```python
from build123d import *

# Parameters (mm, degrees)
ESBO_O2_W                = 8
ESBO_O2_H                = 12
RESSALTO_EXTRUS_O1_DEPTH = 17
ESBO_O3_W                = 6.2
ESBO_O3_H                = 10.2
CORTE_EXTRUS_O1_DEPTH    = 15
ESBO_O4_R                = 12.5
RESSALTO_EXTRUS_O2_DEPTH = 12
ESBO_O5_R                = 11.5
CORTE_EXTRUS_O2_DEPTH    = 10


with BuildPart() as part:
    # Esboço2 → Ressalto-extrusão1 (new body)
    with BuildSketch(Plane.XY):
        Rectangle(ESBO_O2_W, ESBO_O2_H)
    extrude(amount=RESSALTO_EXTRUS_O1_DEPTH)

    # Esboço3 → Corte-extrusão1 (cut)
    with BuildSketch(Plane.XY.offset(17)):
        Rectangle(ESBO_O3_W, ESBO_O3_H)
    extrude(amount=-CORTE_EXTRUS_O1_DEPTH, mode=Mode.SUBTRACT)

    # Esboço4 → Ressalto-extrusão2 (add)
    with BuildSketch(Plane(origin=(0, 6, 0), x_dir=(1, 0, 0), z_dir=(0, 1, 0))):
        with Locations((0, 11.842719282)):
            Circle(ESBO_O4_R)
    extrude(amount=-RESSALTO_EXTRUS_O2_DEPTH)

    # Esboço5 → Corte-extrusão2 (cut)
    with BuildSketch(Plane(origin=(0, 6, 0), x_dir=(1, 0, 0), z_dir=(0, 1, 0))):
        with Locations(Location((0, 11.842719282, 0), (0, 0, 180))):
            Circle(ESBO_O5_R)
    extrude(amount=-CORTE_EXTRUS_O2_DEPTH, mode=Mode.SUBTRACT)


solid = part.part
```
Check sheet for the modelled part. Datum: model origin and axes. Units: mm. A direction names the side the tool comes from. Give positions to 0.01 mm unless a question says otherwise; leave off trailing zeros. Write each loop counter-clockwise with the first axis right and the second up, starting at its lowest first coordinate (ties: lowest second). Pieces come first, ordered by that corner, then holes. Notation, with made-up numbers: (75.5, 55.25) - (97.5, 55.25) arc R18 cw to (97.5, 77.25) - close; hole circle Ø3 at (39, 68.5). An arc over 180 degrees is marked (long way). Answer as a JSON object with one key per item and string values. Group by question number.
1) Release check for a two-part mould opening along X. For faces 1 (the face through (0.493, 0.084, -24.333)), 2 (the face through (4, 0, 8)), 3 (the face through (0, 6, 2)), 4 (the face through (-3.1, 0, 10)) record: pulls with the +X half, pulls with the -X half, needs draft (parallel to the pull), parting line crosses it, or undercut.
2) Sectioned sample at B-B (y = 0). Record the cut outline in (x, z), then the cut area to 3 significant figures.
3) Sectioned sample at D-D (z = -15). Record the cut outline in (x, y).
4) Access from +Z, -Z, +X, -X, +Y, -Y to the whole of each face (thin tool, end or side, straight path). Record for faces 5 (the face through (-4, 0, 8)), 6 (the face through (0, -6, -9)), 7 (the face through (0, 5.1, 10)), 8 (the face through (0, -4, -12)), 9 (the face through (3.5, 0.1, 17)).
5) Sectioned sample at C-C (x = -4.5). Record the cut outline in (y, z), then the cut area to 3 significant figures.
6) Thickness scan on probe 1 along Y at (x, z) = (-2.75, 13); probe 2 along Z at (x, y) = (0, 2.75); probe 3 along X at (y, z) = (0.75, 4). Record the ranges inside material, lowest first. Write a range as from..to.
7) Sectioned sample at A-A (z = 3). Record the cut outline in (x, y).
8) Depth check by flat-ended pin: P1, Ø3, axis at y = -2, z = 7, coming from the +X side; P2, Ø4, axis at x = -4, z = -14.5, coming from the +Y side; P3, Ø5, axis at x = 4, y = 0.5, coming from the -Z side. Enter the tip coordinate at first touch or a pass-through.
Geometry results:
{
 "1": {"face 1": "parting line crosses it", "face 2": "pulls with the +X half", "face 3": "needs draft", "face 4": "undercut"},
 "2": {"outline": "(-4, 0) arc R12.5 ccw (long way) to (4, 0) - (4, 17) - (3.1, 17) - (3.1, 2) - (-3.1, 2) - (-3.1, 17) - (-4, 17) - close; hole circle Ø23 at (0, -11.84)", "area": "115 mm^2"},
 "3": {"outline": "(-12.09, -6) - (12.09, -6) - (12.09, 6) - (11.06, 6) - (11.06, -4) - (-11.06, -4) - (-11.06, 6) - (-12.09, 6) - close"},
 "4": {"face 5": "+Z, -X, +Y, -Y", "face 6": "+Z, -Z, +X, -X, -Y", "face 7": "+Z", "face 8": "+Y", "face 9": "+Z, +X, -X, +Y, -Y"},
 "5": {"outline": "(-6, -23.5) - (6, -23.5) - (6, -22.43) - (-4, -22.43) - (-4, -1.26) - (6, -1.26) - (6, -0.18) - (-6, -0.18) - close", "area": "68.2 mm^2"},
 "6": {"probe 1": "y = -6..-5.1, 5.1..6", "probe 2": "z = -24.34..-23.34, -0.34..2", "probe 3": "x = -4..-3.1, 3.1..4"},
 "7": {"outline": "(-4, -6) - (4, -6) - (4, 6) - (-4, 6) - close; hole (-3.1, -5.1) - (3.1, -5.1) - (3.1, 5.1) - (-3.1, 5.1) - close"},
 "8": {"P1": "stops at x = 4", "P2": "stops at y = -4", "P3": "stops at z = -24.25"}
}
